Design review of the part shown in the three views and the two pictorial views. Dimensions are in mm from the part's minimum x, y and z. A direction names the side the tool comes from. Round coordinates to 2 decimals unless told otherwise and drop trailing zeros. Write each loop counter-clockwise with the first axis right and the second up, starting at its lowest first coordinate (ties: lowest second). Pieces come first, ordered by that corner, then holes. Notation, with made-up numbers: (30, -34.5) -> (50, -34.5) arc R21 cw to (50, 1.5) -> close; hole circle Ø2 at (14.5, 20.5). An arc over 180 degrees is marked (long way). Return JSON: item names as keys, results as strings. Group by question number.
1. For line 1 along X through (y, z) = (7.5, 17); line 2 along Z through (x, y) = (13, 26); line 3 along Z through (x, y) = (0.95, 20), list the stretches that pass through material, from the lowest coordinate up. Write a range as from..to.
2. Take a section at B-B, the plane y = 20. Write out the cut boundary in (x, z).
3. Take a section at D-D, the plane x = 24. Write out the cut boundary in (y, z).
4. Take a section at C-C, the plane z = 40.5. Write out the cut boundary in (x, y).
5. Clearance check with flat-ended pins moving along their axes: P1, Ø13.5, axis at y = 20, z = 44.63, coming from the +X side; P2, Ø4, axis at x = 30.5, y = 9, coming from the +Z side. State where each tip first meets the part, or that it passes through.
6. Take a section at A-A, the plane z = 9. Write out the cut boundary in (x, y).
7. Tool access review of the marked faces 1 and 2: name each direction out of +Z, -Z, +X, -X, +Y, -Y from which nothing blocks a thin tool from reaching the whole face with its end or side.
8. Mouldability with a two-part tool opening along X and no side actions: class the marked faces 3, 4, 5 and 6 as pulls with the +X half, pulls with the -X half, needs draft (parallel to the pull), parting line crosses it, or undercut.
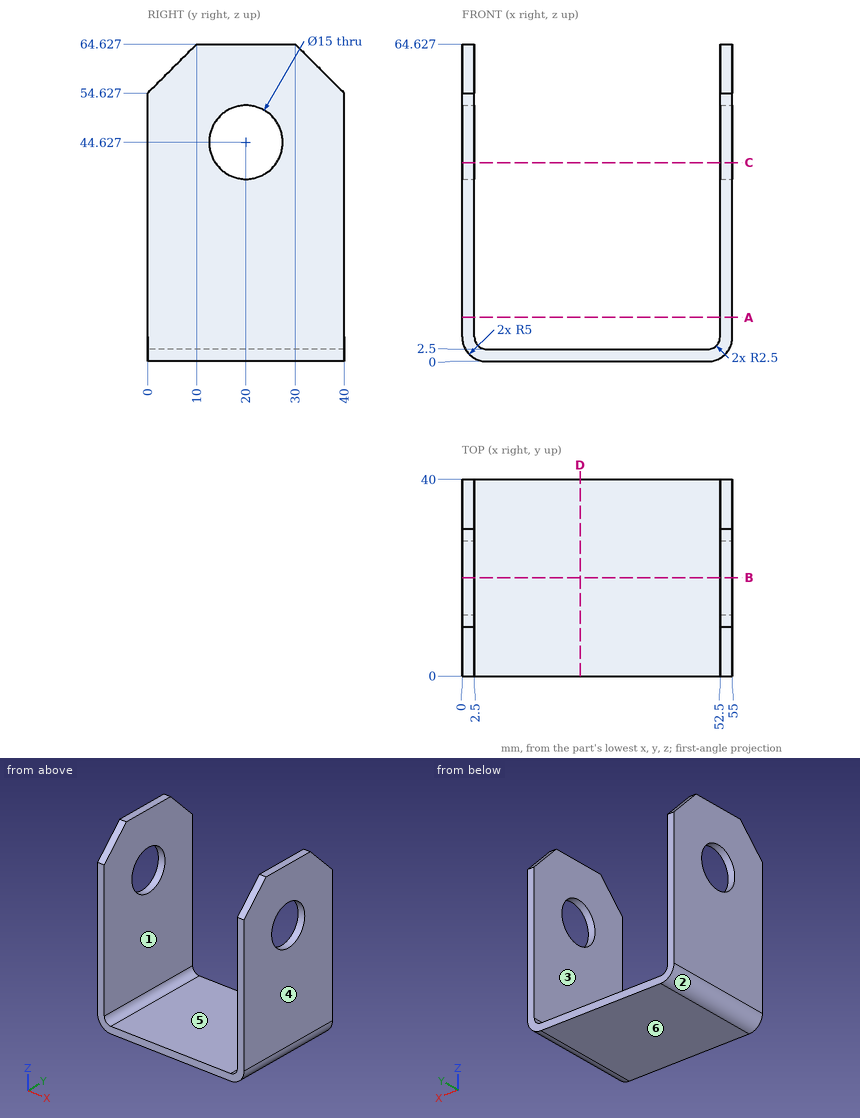
Output:
{
 "1": {"line 1": "x = 0..2.5, 52.5..55", "line 2": "z = 0..2.5", "line 3": "z = 2.07..37.13, 52.13..64.63"},
 "2": {"outline": "(0, 5) arc R5 ccw to (5, 0) -> (50, 0) arc R5 ccw to (55, 5) -> (55, 37.13) -> (52.5, 37.13) -> (52.5, 5) arc R2.5 cw to (50, 2.5) -> (5, 2.5) arc R2.5 cw to (2.5, 5) -> (2.5, 37.13) -> (0, 37.13) -> close; (0, 52.13) -> (2.5, 52.13) -> (2.5, 64.63) -> (0, 64.63) -> close; (52.5, 52.13) -> (55, 52.13) -> (55, 64.63) -> (52.5, 64.63) -> close"},
 "3": {"outline": "(0, 0) -> (40, 0) -> (40, 2.5) -> (0, 2.5) -> close"},
 "4": {"outline": "(0, 0) -> (2.5, 0) -> (2.5, 13.74) -> (0, 13.74) -> close; (0, 26.26) -> (2.5, 26.26) -> (2.5, 40) -> (0, 40) -> close; (52.5, 0) -> (55, 0) -> (55, 13.74) -> (52.5, 13.74) -> close; (52.5, 26.26) -> (55, 26.26) -> (55, 40) -> (52.5, 40) -> close"},
 "5": {"P1": "passes through", "P2": "stops at z = 2.5"},
 "6": {"outline": "(0, 0) -> (2.5, 0) -> (2.5, 40) -> (0, 40) -> close; (52.5, 0) -> (55, 0) -> (55, 40) -> (52.5, 40) -> close"},
 "7": {"face 1": "+Z, +Y, -Y", "face 2": "-Z, -X, +Y, -Y"},
 "8": {"face 3": "undercut", "face 4": "pulls with the +X half", "face 5": "undercut", "face 6": "needs draft"}
}
